Part print with two shaded views. Sizes in mm from the minimum x, y, z corner. A direction names the side the tool comes from. Round coordinates to 2 decimals unless told otherwise and drop trailing zeros. Loops run counter-clockwise (first coordinate to the right, second up) from the corner with the lowest first, then second, coordinate; pieces in that order, holes last. Notation, with made-up numbers: (63, 73) - (116, 73) arc R7 cw to (116, 82) - close; hole circle Ø6 at (53, 84.5). An arc over 180 degrees is marked (long way). Put each result on its own line as item: value. Start each with the question number.
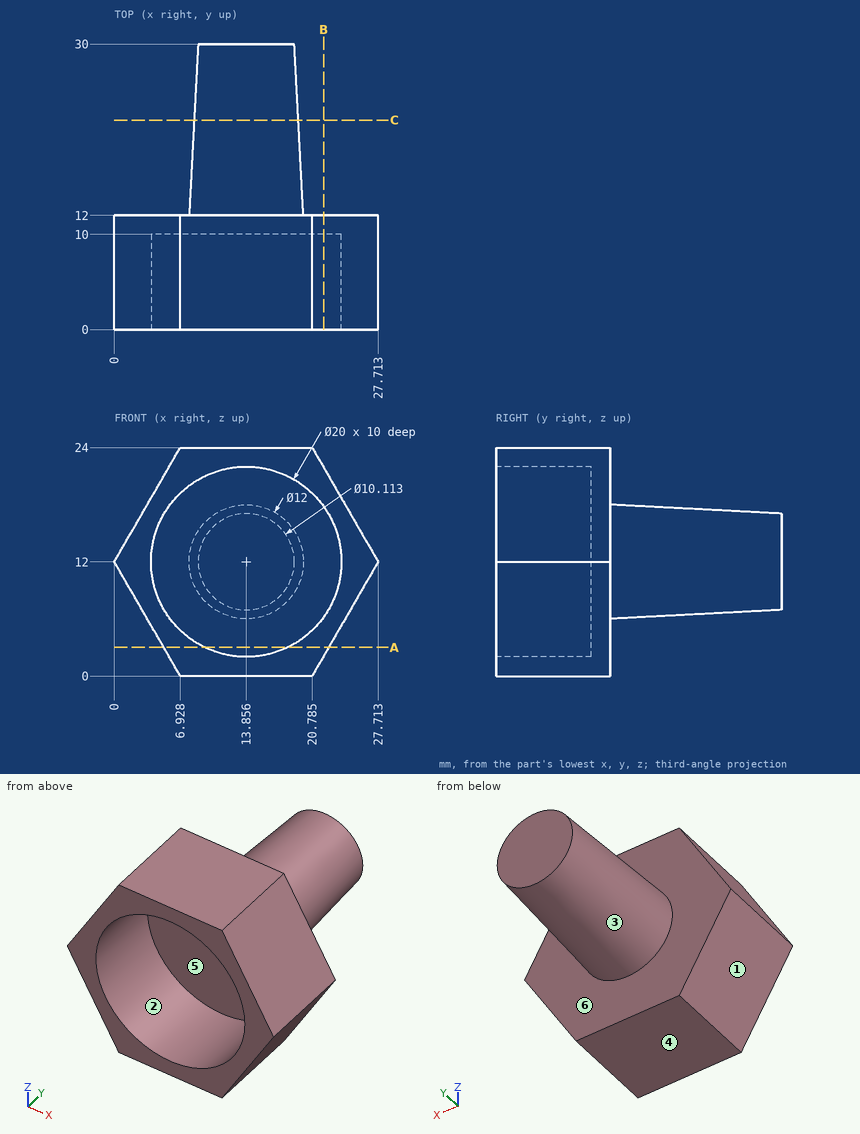
1) Slice it at C-C, the plane y = 22. Write the cut outline in (x, z).
2) Slice it at B-B, the plane x = 22. Write the cut outline in (y, z) (1 decimal).
3) Drop flat-ended pins along their axis: pin 1 Ø12 at (x, y) = (9, 23) entering from +Z; pin 2 Ø10 at (x, z) = (13.5, 10.5) entering from -Y; pin 3 Ø2 at (y, z) = (3.5, 7.5) entering from +X. Give the stop position or say it passes through.
4) Drill centre lines: line 1 (X direction, y = 6.25, z = 12) (1 decimal); line 2 (Y direction, x = 18, z = 14.75); line 3 (Y direction, x = 3, z = 8). Where is each one in solid material? Low to high. Write a range as [from, to].
5) Slice it at A-A, the plane z = 3. Write the cut outline in (x, y) (1 decimal), and give its area (3 significant figures).
6) Pull direction X, two halves, no side cores. Call the marked faces 1, 2 and 3: pulls with the +X half, pulls with the -X half, needs draft (parallel to the pull), parting line crosses it, or undercut.
7) Which spindle directions (+Z, -Z, +X, -X, +Y, -Y) get a long thin tool onto all of the face, cutting with end or side? Do the marked faces 4, 5 and 6. Say none if no direction does.
Taken from the geometry:
1. outline: circle Ø10.95 at (13.86, 12)
2. outline: (0, 2.1) - (12, 2.1) - (12, 21.9) - (0, 21.9) - (0, 17.8) - (10, 17.8) - (10, 6.2) - (0, 6.2) - close
3. pin 1: stops at z = 17.62
3. pin 2: stops at y = 10
3. pin 3: stops at x = 25.69
4. line 1: x = [0, 3.9], [23.9, 27.7]
4. line 2: y = [10, 30]
4. line 3: y = [0, 12]
5. outline: (5.2, 0) - (9.5, 0) - (9.5, 10) - (18.2, 10) - (18.2, 0) - (22.5, 0) - (22.5, 12) - (5.2, 12) - close
5. area: 121 mm2
6. face 1: pulls with the -X half
6. face 2: undercut
6. face 3: parting line crosses it
7. face 4: -Z, +X, -X, +Y, -Y
7. face 5: -Y
7. face 6: +Y
